Drawing for the job (mm, zero at the part's lowest x, y, z). Round coordinates to 2 decimals unless told otherwise and drop trailing zeros. Write each loop counter-clockwise with the first axis right and the second up, starting at its lowest first coordinate (ties: lowest second). Pieces come first, ordered by that corner, then holes.
Item 1: Band-saw the part on D-D, the plane z = 40. Write the cut outline in (x, y).
Item 2: Wall check: probe 1 along X at (y, z) = (4.25, 70); probe 2 along X at (y, z) = (7.8, 40); probe 3 along Z at (x, y) = (19.5, 1.75). Give the ranges that are in metal, low to high.
Item 3: Drop flat-ended pins along their axis: pin 1 Ø5 at (x, z) = (40, 70) entering from +Y; pin 2 Ø12 at (x, z) = (6, 23) entering from -Y; pin 3 Ø3 at (x, z) = (41.5, 41) entering from -Y. Give the stop position or say it passes through.
Item 4: Band-saw the part on B-B, the plane y = 2.25. Write the cut outline in (x, z).
Item 5: Band-saw the part on C-C, the plane y = 7.5. Write the cut outline in (x, z), then the cut area to 3 significant figures.
Item 6: Mould opens along Z. For the marked faces 1, 2, 3 and 4 say: +Z half, -Z half, draft (parallel to the pull), parting line (faces both ways), or undercut.
Item 7: Band-saw the part on A-A, the plane x = 16. Write the cut outline in (y, z), then the cut area to 3 significant figures.
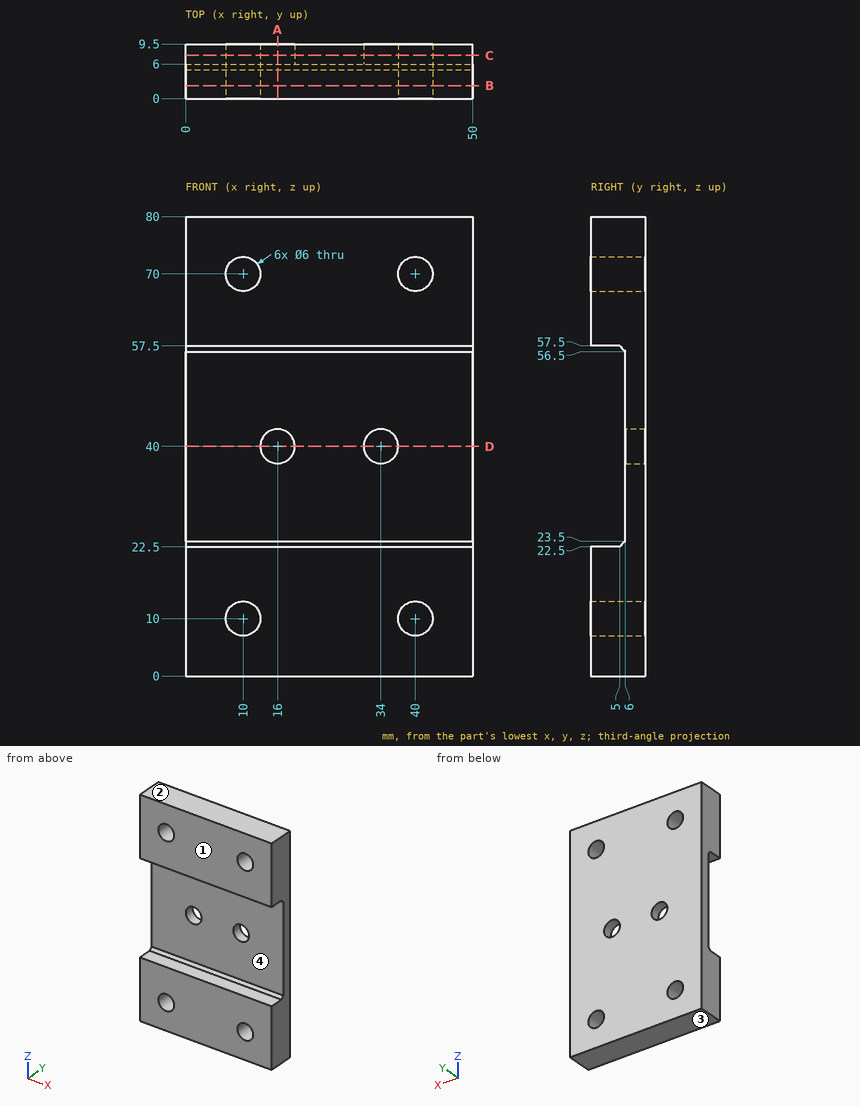
Results:
1. outline: (0, 6) - (13, 6) - (13, 9.5) - (0, 9.5) - close; (19, 6) - (31, 6) - (31, 9.5) - (19, 9.5) - close; (37, 6) - (50, 6) - (50, 9.5) - (37, 9.5) - close
2. probe 1: x = 0 to 7, 13 to 37, 43 to 50
2. probe 2: x = 0 to 13, 19 to 31, 37 to 50
2. probe 3: z = 0 to 22.5, 57.5 to 80
3. pin 1: passes through
3. pin 2: stops at y = 0
3. pin 3: stops at y = 6
4. outline: (0, 0) - (50, 0) - (50, 22.5) - (0, 22.5) - close; (0, 57.5) - (50, 57.5) - (50, 80) - (0, 80) - close; hole circle Ø6 at (10, 10); hole circle Ø6 at (10, 70); hole circle Ø6 at (40, 10); hole circle Ø6 at (40, 70)
5. outline: (0, 0) - (50, 0) - (50, 80) - (0, 80) - close; hole circle Ø6 at (10, 10); hole circle Ø6 at (10, 70); hole circle Ø6 at (16, 40); hole circle Ø6 at (34, 40); hole circle Ø6 at (40, 10); hole circle Ø6 at (40, 70)
5. area: 3,830 mm2
6. face 1: draft
6. face 2: +Z half
6. face 3: -Z half
6. face 4: undercut
7. outline: (0, 0) - (9.5, 0) - (9.5, 37) - (6, 37) - (6, 23.5) - (5, 22.5) - (0, 22.5) - close; (0, 57.5) - (5, 57.5) - (6, 56.5) - (6, 43) - (9.5, 43) - (9.5, 80) - (0, 80) - close
7. area: 530 mm2
